Part model, mm, in its own coordinate system. Face numbers are marked on the shaded views. A direction names the side the tool comes from. Give positions to 0.01 mm unless a question says otherwise; leave off trailing zeros. Write each loop counter-clockwise with the first axis right and the second up, starting at its lowest first coordinate (ties: lowest second). Pieces come first, ordered by that corner, then holes. Notation, with made-up numbers: M 59,44.25 L 68,44.25 A26 cw 68,76.25 Z; hole C 81.5,79 d1. An arc over 180 degrees is marked long. Write item = value, one per line. Start each with the question number.
from build123d import *

# Parameters (mm, degrees)
SKETCH1_R           = 4
SKETCH1_R_2         = 1.5
BOSS_EXTRUDE1_DEPTH = 3
CHAMFER1_SIZE       = 0.8


with BuildPart() as part:
    # Sketch1 → Boss-Extrude1 (new body)
    with BuildSketch(Plane(origin=(0, 0, 0), x_dir=(1, 0, 0), z_dir=(0, 1, 0))):
        with BuildLine():
            Line((-3.5, 17.25), (-3.5, 8.5))
            ThreePointArc((-3.5, 8.5), (-4.964466094, 4.964466094), (-8.5, 3.5))
            Line((-8.5, 3.5), (-17.25, 3.5))
            ThreePointArc((-17.25, 3.5), (-20.75, 0), (-17.25, -3.5))
            Line((-17.25, -3.5), (-8.5, -3.5))
            ThreePointArc((-8.5, -3.5), (-4.964466094, -4.964466094), (-3.5, -8.5))
            Line((-3.5, -8.5), (-3.5, -17.25))
            ThreePointArc((-3.5, -17.25), (0, -20.75), (3.5, -17.25))
            Line((3.5, -17.25), (3.5, -8.5))
            ThreePointArc((3.5, -8.5), (4.964466094, -4.964466094), (8.5, -3.5))
            Line((8.5, -3.5), (17.25, -3.5))
            ThreePointArc((17.25, -3.5), (20.75, 0), (17.25, 3.5))
            Line((17.25, 3.5), (8.5, 3.5))
            ThreePointArc((8.5, 3.5), (4.964466094, 4.964466094), (3.5, 8.5))
            Line((3.5, 8.5), (3.5, 17.25))
            ThreePointArc((3.5, 17.25), (0, 20.75), (-3.5, 17.25))
        make_face()
        Circle(SKETCH1_R, mode=Mode.SUBTRACT)
        with Locations((0, 17.25)):
            Circle(SKETCH1_R_2, mode=Mode.SUBTRACT)
        with Locations((17.25, 0)):
            Circle(SKETCH1_R_2, mode=Mode.SUBTRACT)
        with Locations((0, -17.25)):
            Circle(SKETCH1_R_2, mode=Mode.SUBTRACT)
        with Locations((-17.25, 0)):
            Circle(SKETCH1_R_2, mode=Mode.SUBTRACT)
        with Locations((-8, 0)):
            Circle(SKETCH1_R_2, mode=Mode.SUBTRACT)
        with Locations((8, 0)):
            Circle(SKETCH1_R_2, mode=Mode.SUBTRACT)
        with Locations((0, 9.5)):
            Circle(SKETCH1_R_2, mode=Mode.SUBTRACT)
        with Locations((0, -9.5)):
            Circle(SKETCH1_R_2, mode=Mode.SUBTRACT)
    extrude(amount=BOSS_EXTRUDE1_DEPTH)

    # Chamfer1
    chamfer1_edges = [part.edges().sort_by_distance(p)[0] for p in [
        (-9.5, 3, 0),
        (6.5, 3, 0),
        (-1.5, 3, -9.5),
        (-1.5, 3, 9.5),
    ]]
    chamfer(chamfer1_edges, length=CHAMFER1_SIZE)


solid = part.part
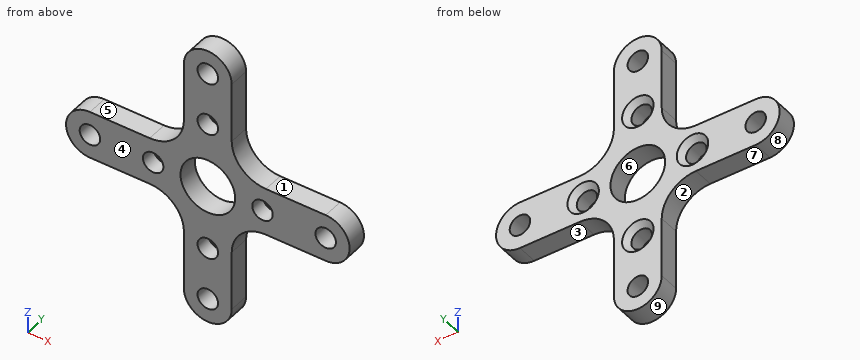
Q1. Two-plate mould, pull along X, no slides. Class the marked faces 6, 7, 8 and 9: +X half, -X half, draft (parallel to the pull), parting line (faces both ways), or undercut.
Q2. Slice it at C-C (z = 0). Give the cut face in (x, y).
Q3. Slice it at A-A (z = 9.5). Give the cut face in (x, y), and give its area (3 significant figures).
Q4. Slice it at D-D (x = 16.5). Give the cut face in (y, z).
Q5. Slice it at B-B (x = 0). Give the cut face in (y, z).
Q6. Probe line 1 along Z through (x, y) = (0, 1.1); line 2 along X through (y, z) = (1.7, 0); line 3 along X through (y, z) = (0.6, 9.5). List the from-to ranges inside material, lowest first.
Q7. Tool access for the marked faces 1, 2, 3, 4 and 5: list every direction of +Z, -Z, +X, -X, +Y, -Y with a clear straight run to the whole face (end or side of a thin tool).
Q8. Drop flat-ended pins along their axis: P1, Ø0.9, axis at x = 12, y = 1.5, coming from the +Z side; P2, Ø0.9, axis at y = 2, z = 11, coming from the -X side; P3, Ø1.5, axis at y = 2, z = 14, coming from the +X side. Give the stop position or say it passes through.
Working result:
q1.face_6 = undercut
q1.face_7 = draft
q1.face_8 = -X half
q1.face_9 = parting line
q2.outline = M -20.75,0 L -18.75,0 L -18.75,3 L -20.75,3 Z; M -15.75,0 L -9.5,0 L -9.5,2.2 L -10.3,3 L -15.75,3 Z; M -6.5,0 L -4,0 L -4,3 L -5.7,3 L -6.5,2.2 Z; M 4,0 L 6.5,0 L 6.5,2.2 L 5.7,3 L 4,3 Z; M 9.5,0 L 15.75,0 L 15.75,3 L 10.3,3 L 9.5,2.2 Z; M 18.75,0 L 20.75,0 L 20.75,3 L 18.75,3 Z
q3.outline = M -3.5,0 L -1.5,0 L -1.5,2.2 L -2.3,3 L -3.5,3 Z; M 1.5,0 L 3.5,0 L 3.5,3 L 2.3,3 L 1.5,2.2 Z
q3.area = 11.4 mm2
q4.outline = M 0,-3.5 L 3,-3.5 L 3,-1.3 L 0,-1.3 Z; M 0,1.3 L 3,1.3 L 3,3.5 L 0,3.5 Z
q5.outline = M 0,-20.75 L 3,-20.75 L 3,-18.75 L 0,-18.75 Z; M 0,-15.75 L 3,-15.75 L 3,-11.8 L 2.2,-11 L 0,-11 Z; M 0,-8 L 2.2,-8 L 3,-7.2 L 3,-4 L 0,-4 Z; M 0,4 L 3,4 L 3,7.2 L 2.2,8 L 0,8 Z; M 0,11 L 2.2,11 L 3,11.8 L 3,15.75 L 0,15.75 Z; M 0,18.75 L 3,18.75 L 3,20.75 L 0,20.75 Z
q6.line_1 = -20.75 to -18.75, -15.75 to -11, -8 to -4, 4 to 8, 11 to 15.75, 18.75 to 20.75
q6.line_2 = -20.75 to -18.75, -15.75 to -9.5, -6.5 to -4, 4 to 6.5, 9.5 to 15.75, 18.75 to 20.75
q6.line_3 = -3.5 to -1.5, 1.5 to 3.5
q7.face_1 = +Z, +X, +Y, -Y
q7.face_2 = -Z, -X, +Y, -Y
q7.face_3 = -Z, +X, +Y, -Y
q7.face_4 = +Z, -Z, +X, -X, -Y
q7.face_5 = +Z, -X, +Y, -Y
q8.P1 = 3.5
q8.P2 = -3.5
q8.P3 = 3.5
